Part model, mm, in its own coordinate system. A direction names the side the tool comes from. Round coordinates to 2 decimals unless told otherwise and drop trailing zeros.
(1) Tool access for faces 3 (the face through (17, -3, 25.4)), 4 (the face through (-2.13, 16.25, 16.63)): list every direction of +Z, -Z, +X, -X, +Y, -Y with a clear straight run to the whole face (end or side of a thin tool).
(2) Mould opens along Y. For faces 1 (the face through (1, 1, 0)), 2 (the face through (0, 0, 7.62)) say: +Y half, -Y half, draft (parallel to the pull), parting line (faces both ways), or undercut.
(3) Flat gauge pins, fed straight in: pin 1 (5 mm diameter, centred on x = 2.5, z = 6, fed in from +Y); pin 2 (1.5 mm diameter, centred on y = -10.5, z = 19, fed in from -X); pin 3 (12 mm diameter, centred on y = -3.5, z = 6.5, fed in from +X). Where does each tip first touch, or does it go through?
(4) Probe probe 1 along Z at (x, y) = (6, 11.5); probe 2 along Y at (x, z) = (0, 13); probe 3 along Y at (x, z) = (-5, 14.75). List the from-to ranges inside material, lowest first.
from build123d import *

# Parameters (mm, degrees)
F4_R     = 16.3873393924
F5_DEPTH = 17.78


# Not quite as in the source:
# - the arcs of a loft's sections are written as splines that run evenly, so that the points pair up as in the source's solid


with BuildPart() as f3:
    # F1 (on Top) → F3 section 0
    with BuildSketch(Plane.XY):
        with BuildLine():
            add(Edge.make_bspline(
                [(43.2906929066, 2.1420251998), (43.1660749319, 4.6605756221), (42.821117674, 7.168184659), (41.7009847964, 12.0854812551), (40.9258264748, 14.495092877), (38.9688313396, 19.1431756557), (37.7870247476, 21.3815750327), (35.0526296616, 25.6192143509), (33.5000833946, 27.6183888507), (30.071371569, 31.3168261821), (28.1952589595, 33.0160318991), (24.176410068, 36.0628920967), (22.0337358485, 37.4104995251), (17.546860581, 39.7132052837), (15.2027288233, 40.6682680536), (10.3841586143, 42.156852824), (7.9097945757, 42.6903518365), (2.9059392428, 43.3195857237), (0.3765252225, 43.4153108812), (-4.6605756221, 43.1660749319), (-7.168184659, 42.821117674), (-12.0854812551, 41.7009847964), (-14.495092877, 40.9258264748), (-19.1431756557, 38.9688313396), (-21.3815750327, 37.7870247476), (-23.5003946918, 36.4198272046)],
                knots=[0, 0, 0, 0, 0.0833333333, 0.0833333333, 0.1666666667, 0.1666666667, 0.25, 0.25, 0.3333333333, 0.3333333333, 0.4166666667, 0.4166666667, 0.5, 0.5, 0.5833333333, 0.5833333333, 0.6666666667, 0.6666666667, 0.75, 0.75, 0.8333333333, 0.8333333333, 0.9166666667, 0.9166666667, 1, 1, 1, 1], degree=3))
            add(Edge.make_bspline(
                [(-23.5003946918, 36.4198272046), (-25.6192143509, 35.0526296616), (-27.6183888507, 33.5000833946), (-31.3168261821, 30.071371569), (-33.0160318991, 28.1952589595), (-36.0628920967, 24.176410068), (-37.4104995251, 22.0337358485), (-39.7132052837, 17.546860581), (-40.6682680536, 15.2027288233), (-42.156852824, 10.3841586143), (-42.6903518365, 7.9097945757), (-43.3195857237, 2.9059392428), (-43.4153108812, 0.3765252225), (-43.1660749319, -4.6605756221), (-42.821117674, -7.168184659), (-41.7009847964, -12.0854812551), (-40.9258264748, -14.495092877), (-38.9688313396, -19.1431756557), (-37.7870247476, -21.3815750327), (-35.0526296616, -25.6192143509), (-33.5000833946, -27.6183888507), (-30.071371569, -31.3168261821), (-28.1952589595, -33.0160318991), (-24.176410068, -36.0628920967), (-22.0337358485, -37.4104995251), (-19.7902982147, -38.5618524044)],
                knots=[0, 0, 0, 0, 0.0833333333, 0.0833333333, 0.1666666667, 0.1666666667, 0.25, 0.25, 0.3333333333, 0.3333333333, 0.4166666667, 0.4166666667, 0.5, 0.5, 0.5833333333, 0.5833333333, 0.6666666667, 0.6666666667, 0.75, 0.75, 0.8333333333, 0.8333333333, 0.9166666667, 0.9166666667, 1, 1, 1, 1], degree=3))
            add(Edge.make_bspline(
                [(-19.7902982147, -38.5618524044), (-17.546860581, -39.7132052837), (-15.2027288233, -40.6682680536), (-10.3841586143, -42.156852824), (-7.9097945757, -42.6903518365), (-2.9059392428, -43.3195857237), (-0.3765252225, -43.4153108812), (4.6605756221, -43.1660749319), (7.168184659, -42.821117674), (12.0854812551, -41.7009847964), (14.495092877, -40.9258264748), (19.1431756557, -38.9688313396), (21.3815750327, -37.7870247476), (25.6192143509, -35.0526296616), (27.6183888507, -33.5000833946), (31.3168261821, -30.071371569), (33.0160318991, -28.1952589595), (36.0628920967, -24.176410068), (37.4104995251, -22.0337358485), (39.7132052837, -17.546860581), (40.6682680536, -15.2027288233), (42.156852824, -10.3841586143), (42.6903518365, -7.9097945757), (43.3195857237, -2.9059392428), (43.4153108812, -0.3765252225), (43.2906929066, 2.1420251998)],
                knots=[0, 0, 0, 0, 0.0833333333, 0.0833333333, 0.1666666667, 0.1666666667, 0.25, 0.25, 0.3333333333, 0.3333333333, 0.4166666667, 0.4166666667, 0.5, 0.5, 0.5833333333, 0.5833333333, 0.6666666667, 0.6666666667, 0.75, 0.75, 0.8333333333, 0.8333333333, 0.9166666667, 0.9166666667, 1, 1, 1, 1], degree=3))
        make_face()
    # F2 (on offset) → F3 section 1
    with BuildSketch(Plane.XY.offset(25.4)):
        Polygon((47.3345444493, 2.3421151343), (-25.6956034295, 39.8218604025), (-21.6389410198, -42.1639755368), align=None)
    loft(ruled=True)

    # F4 (on face) → F5 (cut)
    with BuildSketch(Plane.XY.offset(25.4)):
        Circle(F4_R)
    extrude(amount=-F5_DEPTH, mode=Mode.SUBTRACT)


solid = f3.part
Final values:
1. face 3: +Z, +X, -X, +Y, -Y
1. face 4: +Z
2. face 1: draft
2. face 2: undercut
3. pin 1: stops at y = 41.17
3. pin 2: stops at x = -28.44
3. pin 3: stops at x = 44.65
4. probe 1: z = 0 to 7.62
4. probe 2: y = -36.63 to -16.39, 16.39 to 35.55
4. probe 3: y = -37.29 to -15.61, 15.61 to 35.78
